from build123d import *

# Parameters (mm, degrees)
CIRPATTERN1_COUNT = 3


with BuildPart() as part:
    # Sketch1 → Revolve1 (revolve)
    with BuildSketch(Plane.XY, mode=Mode.PRIVATE) as revolve1_sk:
        Polygon((0, 14.478), (21.149404438, 14.478), (21.149404438, 15.9385), (29.404404438, 15.9385), (29.404404438, 15.494), (3.81, 8.636), (3.81, 10.16), (0, 10.16), align=None)
    revolve(revolve1_sk.sketch.rotate(Axis((0, 0, 0), (1, 0, 0)), 90), axis=Axis((0, 0, 0), (1, 0, 0)))

    # Sketch3 → #6-32 Tapped Hole1 (revolve, cut)
    with BuildSketch(Plane(origin=(3.369404438, 14.478, 0), x_dir=(0, 0, 1), z_dir=(1, 0, 0))):
        Polygon((0, 0), (0, 4.445), (1.35255, 3.63230597), (1.35255, 0), align=None)
    f_6_32_tapped_hole1 = revolve(axis=Axis((3.369404438, 20.828, 0), (0, -1, 0)), mode=Mode.SUBTRACT)

    # CirPattern1: #6-32 Tapped Hole1 ×3 about axis
    cirpattern1_axis = Axis((0, 0, 0), (-1, 0, 0))
    for i in range(1, CIRPATTERN1_COUNT):
        add(f_6_32_tapped_hole1.rotate(cirpattern1_axis, i * 360 / CIRPATTERN1_COUNT), mode=Mode.SUBTRACT)


solid = part.part
The listing builds one solid part. Answer for the finished solid, in the listing's coordinates (mm). A direction names the side the tool comes from. Coordinates: 2 decimals unless noted, no trailing zeros. Write each loop counter-clockwise with the first axis right and the second up, starting at its lowest first coordinate (ties: lowest second). Pieces come first, ordered by that corner, then holes. Notation, with made-up numbers: (45.5, 76.5) - (95.5, 76.5) arc R37 cw to (95.5, 112.5) - close; hole circle Ø6 at (69, 46). An arc over 180 degrees is marked (long way). Return JSON: item names as keys, results as strings.
1. The part is cut by section A-A on y = 0. Determine the outline of the cut face in (x, z), then the cut area to 3 significant figures.
Final values:
{"outline": "(0, -14.48) - (21.15, -14.48) - (21.15, -15.94) - (29.4, -15.94) - (29.4, -15.49) - (3.81, -8.64) - (3.81, -10.16) - (0, -10.16) - close; (0, 10.16) - (3.81, 10.16) - (3.81, 8.64) - (29.4, 15.49) - (29.4, 15.94) - (21.15, 15.94) - (21.15, 14.48) - (0, 14.48) - close", "area": "181 mm^2"}
2. The part is cut by section C-C on x = 5.25. Determine the outline of the cut face in (y, z), then the cut area to 3 significant figures.
Final values:
{"outline": "circle Ø28.96 at (0, 0); hole circle Ø18.04 at (0, 0)", "area": "403 mm^2"}
3. The part is cut by section B-B on x = 21.75. Determine the outline of the cut face in (y, z), then the cut area to 3 significant figures.
Final values:
{"outline": "circle Ø31.88 at (0, 0); hole circle Ø26.89 at (0, 0)", "area": "230 mm^2"}
4. Consider line 1 along Y through (x, z) = (1.5, 0); line 2 along Z through (x, y) = (4.25, -3); line 3 along Z through (x, y) = (12.75, -9). Determine where each line is inside the solid, lowest interval first.
Final values:
{"line 1": "-14.48 to -10.16, 10.16 to 14.48", "line 2": "-14.16 to -8.22, 8.22 to 14.16", "line 3": "-11.34 to -6.38, 6.38 to 11.34"}
5. For a pull along Y with two mould halves and no side action, classify faces 1 (the face through (0, -10, -3)), 2 (the face through (3.81, 7.5, 4.6)), 3 (the face through (25.3, -4.8, 15.2)) as +Y half, -Y half, draft (parallel to the pull), parting line (faces both ways), or undercut.
Final values:
{"face 1": "draft", "face 2": "undercut", "face 3": "parting line"}
6. Which of the six approach directions +Z, -Z, +X, -X, +Y, -Y give full straight-line access (tool end or side, diameter ignored) to faces 4 (the face through (13.58, 6.85, -8.93)), 5 (the face through (2.03, 12.69, -0.18)), 6 (the face through (1.878, -10.074, -1.323))?
Final values:
{"face 4": "+X", "face 5": "+Y", "face 6": "-X"}
7. Each of these flat-tipped pins is pushed along its axis until it touches: pin 1 Ø8 at (x, z) = (14.5, -8) entering from +Y; pin 2 Ø8 at (y, z) = (-3.5, -4) entering from -X; pin 3 Ø6 at (x, z) = (5, -6.5) entering from -Y. Where does it stop, or does it pass through?
Final values:
{"pin 1": "y = 13.91", "pin 2": "x = 3.81", "pin 3": "y = -14.05"}
